from build123d import *

# Parameters (mm, degrees)
SKETCH1_W                    = 361.95
SKETCH1_H                    = 119.38
BASE_FLANGE1_DEPTH           = 2.65684
EDGE_FLANGE1_STRIP_W         = 16.97736
EDGE_FLANGE1_STRIP_H         = 2.65684
EDGE_FLANGE1_STRIP_CUT_DEPTH = 119.38
EDGE_FLANGE1_DEPTH           = 119.38
EDGE_FLANGE2_STRIP_W         = 16.97736
EDGE_FLANGE2_STRIP_H         = 2.65684
EDGE_FLANGE2_STRIP_CUT_DEPTH = 119.38
EDGE_FLANGE2_DEPTH           = 119.38
SKETCH12_R                   = 6.35
CUT_EXTRUDE1_DEPTH           = 385.85974152


# Sheet-metal steps are written as plain solids
with BuildPart() as part:
    # Sketch1 → Base-Flange1 (new body)
    with BuildSketch(Plane(origin=(0, 0, 0), x_dir=(1, 0, 0), z_dir=(0, 1, 0))):
        with Locations((180.975, 59.69)):
            Rectangle(SKETCH1_W, SKETCH1_H)
    extrude(amount=-BASE_FLANGE1_DEPTH)

    # Edge-Flange1 strip (across the edge) → Edge-Flange1 strip cut (cut)
    with BuildSketch(Plane(origin=(0, -2.65684, 0), x_dir=(1, 0, 0), z_dir=(0, 0, -1))):
        with Locations((-2.65684, -1.32842)):
            Rectangle(EDGE_FLANGE1_STRIP_W, EDGE_FLANGE1_STRIP_H)
    extrude(amount=EDGE_FLANGE1_STRIP_CUT_DEPTH, mode=Mode.SUBTRACT)

    # Edge-Flange1 section (across the edge) → Edge-Flange1 (add)
    with BuildSketch(Plane(origin=(0, -2.65684, 0), x_dir=(1, 0, 0), z_dir=(0, 0, -1))):
        with BuildLine():
            Line((0, 3.175), (0, 50.8))
            Line((0, 50.8), (2.65684, 50.8))
            Line((2.65684, 50.8), (2.65684, 3.175))
            ThreePointArc((2.65684, 3.175), (3.58677597, 0.92993597), (5.83184, 0))
            Line((5.83184, 0), (5.83184, -2.65684))
            ThreePointArc((5.83184, -2.65684), (1.708106389, -0.948733611), (0, 3.175))
        make_face()
    extrude(amount=EDGE_FLANGE1_DEPTH)

    # Edge-Flange2 strip (across the edge) → Edge-Flange2 strip cut (cut)
    with BuildSketch(Plane(origin=(361.95, -2.65684, -119.38), x_dir=(-1, 0, 0), z_dir=(0, 0, 1))):
        with Locations((-2.65684, -1.32842)):
            Rectangle(EDGE_FLANGE2_STRIP_W, EDGE_FLANGE2_STRIP_H)
    extrude(amount=EDGE_FLANGE2_STRIP_CUT_DEPTH, mode=Mode.SUBTRACT)

    # Edge-Flange2 section (across the edge) → Edge-Flange2 (add)
    with BuildSketch(Plane(origin=(361.95, -2.65684, -119.38), x_dir=(-1, 0, 0), z_dir=(0, 0, 1))):
        with BuildLine():
            Line((0, 3.175), (0, 50.8))
            Line((0, 50.8), (2.65684, 50.8))
            Line((2.65684, 50.8), (2.65684, 3.175))
            ThreePointArc((2.65684, 3.175), (3.58677597, 0.92993597), (5.83184, 0))
            Line((5.83184, 0), (5.83184, -2.65684))
            ThreePointArc((5.83184, -2.65684), (1.708106389, -0.948733611), (0, 3.175))
        make_face()
    extrude(amount=EDGE_FLANGE2_DEPTH)

    # Sketch12 → Cut-Extrude1 (cut, through all)
    with BuildSketch(Plane.ZY):
        with Locations(Location((-87.63, -29.64434, 0), (0, 0, 270))):
            Circle(SKETCH12_R)
        with Locations(Location((-31.75, -29.64434, 0), (0, 0, 270))):
            Circle(SKETCH12_R)
    extrude(amount=-CUT_EXTRUDE1_DEPTH, mode=Mode.SUBTRACT)


solid = part.part
Can you work these out from the model? Positions are in its coordinate system, mm. A direction names the side the tool comes from. Give positions to 0.01 mm unless a question says otherwise; leave off trailing zeros. Loops run counter-clockwise (first coordinate to the right, second up) from the corner with the lowest first, then second, coordinate; pieces in that order, holes last. Notation, with made-up numbers: (3.5, 19.25) - (13.5, 19.25) arc R28 cw to (13.5, 58.25) - close; hole circle Ø2 at (44, 10). An arc over 180 degrees is marked (long way). Return JSON: item names as keys, results as strings.
1. I want a section at B-B on y = -43.5. Please give me the cut outline in (x, z), and give its area (3 significant figures).
Output values:
{"outline": "(0, -119.38) - (2.66, -119.38) - (2.66, 0) - (0, 0) - close; (359.29, -119.38) - (361.95, -119.38) - (361.95, 0) - (359.29, 0) - close", "area": "634 mm²"}
2. I want a section at A-A on z = -87.63. Please give me the cut outline in (x, y) (3 decimals), and give its area (3 significant figures).
Output values:
{"outline": "(0, -53.457) - (2.657, -53.457) - (2.657, -35.994) - (0, -35.994) - close; (0, -23.294) - (2.657, -23.294) - (2.657, -5.832) arc R3.175 cw to (5.832, -2.657) - (356.118, -2.657) arc R3.175 cw to (359.293, -5.832) - (359.293, -23.294) - (361.95, -23.294) - (361.95, -5.832) arc R5.832 ccw to (356.118, 0) - (5.832, 0) arc R5.832 ccw to (0, -5.832) - close; (359.293, -53.457) - (361.95, -53.457) - (361.95, -35.994) - (359.293, -35.994) - close", "area": "1,150 mm²"}
3. For faces 1 (the face through (361.95, -29, -61)), 2 (the face through (179, -2.657, -61)), which set-ups out of +Z, -Z, +X, -X, +Y, -Y let a thin tool reach every point of the face, with its end or its side?
Output values:
{"face 1": "+Z, -Z, +X, +Y, -Y", "face 2": "+Z, -Z, -Y"}
4. I want a section at D-D on x = 159.5. Please give me the cut outline in (y, z), and give its area (3 significant figures).
Output values:
{"outline": "(-2.66, -119.38) - (0, -119.38) - (0, 0) - (-2.66, 0) - close", "area": "317 mm²"}
5. I want a section at C-C on z = -41.5. Please give me the cut outline in (x, y) (3 decimals), and give its area (3 significant figures).
Output values:
{"outline": "(0, -53.457) - (2.657, -53.457) - (2.657, -5.832) arc R3.175 cw to (5.832, -2.657) - (356.118, -2.657) arc R3.175 cw to (359.293, -5.832) - (359.293, -53.457) - (361.95, -53.457) - (361.95, -5.832) arc R5.832 ccw to (356.118, 0) - (5.832, 0) arc R5.832 ccw to (0, -5.832) - close", "area": "1,220 mm²"}
6. I'm going to push flat-ended pins straight in: pin 1 Ø10 at (y, z) = (-29.64, -87.63) entering from +X; pin 2 Ø5 at (x, z) = (286.5, -33) entering from -Y. Where does each tip first touch, or does it pass through?
Output values:
{"pin 1": "passes through", "pin 2": "stops at y = -2.66"}
7. If I drill on line 1 (X direction, y = -37.5, z = -17); line 2 (Y direction, x = 255.5, z = -40); line 3 (Y direction, x = 1, z = -31), over which ranges is the centre line in solid material (lowest first)?
Output values:
{"line 1": "x = 0 to 2.66, 359.29 to 361.95", "line 2": "y = -2.66 to 0", "line 3": "y = -53.46 to -35.95, -23.34 to -2.57"}
8. We'd pull the mould along Z, two halves only. Please class faces 3 (the face through (180, -1, -119.38)), 4 (the face through (179, 0, -61)), 5 (the face through (1.31, -28.27, -93.83)), 6 (the face through (360.6, -28.27, -93.83)): +Z half, -Z half, draft (parallel to the pull), parting line (faces both ways), or undercut.
Output values:
{"face 3": "-Z half", "face 4": "draft", "face 5": "undercut", "face 6": "undercut"}
